For this review, take the finished solid that the model builds, in its own axes (mm). Round coordinates to 2 decimals unless told otherwise and drop trailing zeros. Order: outer loops, then holes, each group sorted by start corner. A loop starts at its lowest first (then second) coordinate and runs counter-clockwise, first axis right, second up. Notation, with made-up numbers: (59.5, 24.5) -> (104.5, 24.5) arc R15 cw to (104.5, 29.5) -> close; hole circle Ø2 at (68, 18.25). An arc over 180 degrees is marked (long way). Answer in a Markdown table with one row per item.
```python
from build123d import *

# Parameters (mm, degrees)
SKETCH_R     = 13
PAD_DEPTH    = 70
CHAMFER_SIZE = 40


with BuildPart() as part:
    # Sketch → Pad (new body)
    with BuildSketch(Plane.XZ):
        Polygon((-50, 0), (-190, 0), (-190, 555), (-240, 605), (-240, 890), (0, 890), (0, 605), (-50, 555), align=None)
        with Locations((-120, 635)):
            Circle(SKETCH_R, mode=Mode.SUBTRACT)
    extrude(amount=PAD_DEPTH)

    # Chamfer
    chamfer_edges = [part.edges().sort_by_distance(p)[0] for p in [
        (-120, -70, 890),
        (-120, -70, 0),
    ]]
    chamfer(chamfer_edges, length=CHAMFER_SIZE)


solid = part.part
```
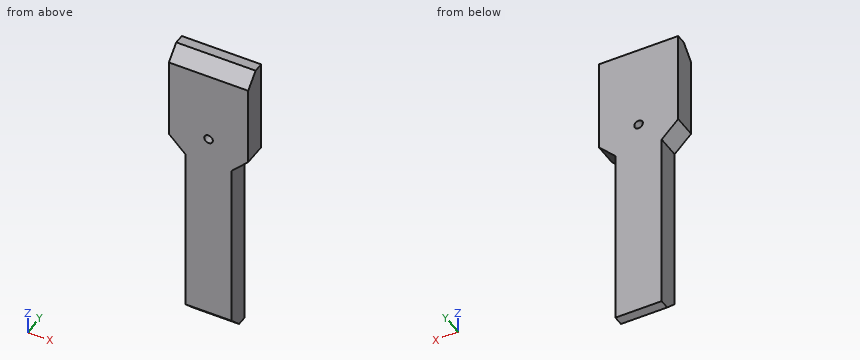
Q1. To check wall thickness, follow probe 1 along X at (y, z) = (-49, 635); probe 2 along Z at (x, y) = (-120, -19); probe 3 along X at (y, z) = (-43, 75). State the ranges of each line that lie inside material, in increasing order.
Answer key:
| item | result |
|---|---|
| probe 1 | x = -240 to -133, -107 to 0 |
| probe 2 | z = 0 to 622, 648 to 890 |
| probe 3 | x = -190 to -50 |
Q2. Take a section at A-A, the plane z = 635. Write out the cut boundary in (x, y).
Answer key:
| item | result |
|---|---|
| outline | (-240, -70) -> (-133, -70) -> (-133, 0) -> (-240, 0) -> close; (-107, -70) -> (0, -70) -> (0, 0) -> (-107, 0) -> close |
Q3. Take a section at D-D, the plane x = -35.5. Write out the cut boundary in (y, z), then the cut area to 3 significant figures.
Answer key:
| item | result |
|---|---|
| outline | (-70, 569.5) -> (0, 569.5) -> (0, 890) -> (-30, 890) -> (-70, 850) -> close |
| area | 21,600 mm^2 |
Q4. Take a section at C-C, the plane y = -41. Write out the cut boundary in (x, z), then the cut area to 3 significant figures.
Answer key:
| item | result |
|---|---|
| outline | (-240, 605) -> (-190, 555) -> (-190, 11) -> (-50, 11) -> (-50, 555) -> (0, 605) -> (0, 879) -> (-240, 879) -> close; hole circle Ø26 at (-120, 635) |
| area | 151,000 mm^2 |
Q5. Clearance check with flat-ended pins moving along their axes: pin 1 Ø21 at (x, z) = (-120, 635) entering from +Y; pin 2 Ø10 at (x, y) = (-56.5, -56.5) entering from +Z; pin 3 Ø1.5 at (y, z) = (-31.5, 223.5) entering from -X; pin 4 Ø21 at (y, z) = (-43, 242) entering from +X. State where each tip first meets the part, or that it passes through.
Answer key:
| item | result |
|---|---|
| pin 1 | passes through |
| pin 2 | stops at z = 868.5 |
| pin 3 | stops at x = -190 |
| pin 4 | stops at x = -50 |
Q6. Take a section at B-B, the plane x = -120. Write out the cut boundary in (y, z).
Answer key:
| item | result |
|---|---|
| outline | (-70, 40) -> (-30, 0) -> (0, 0) -> (0, 622) -> (-70, 622) -> close; (-70, 648) -> (0, 648) -> (0, 890) -> (-30, 890) -> (-70, 850) -> close |
